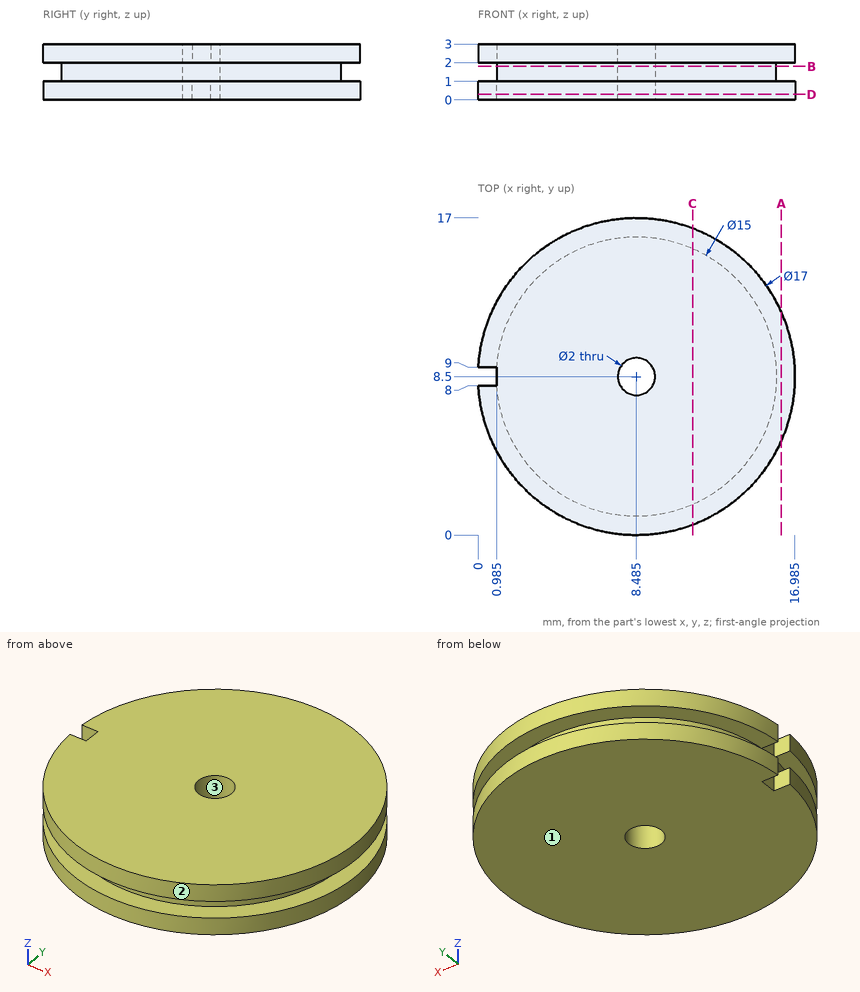
Geometry check sheet. Reference: drawing and pictorial views, mm from the part's lowest x, y, z. Round coordinates to 2 decimals unless told otherwise and drop trailing zeros. Order: outer loops, then holes, each group sorted by start corner. A loop starts at its lowest first (then second) coordinate and runs counter-clockwise, first axis right, second up. Notation, with made-up numbers: (-0.75, 54) - (56.25, 54) arc R29 ccw to (56.25, 86) - close; hole circle Ø3 at (15, 84). An arc over 180 degrees is marked (long way). Use a Markdown table: item, result. Add a question column.
1) Gauge pin test, flat ends, axial feed: P1, Ø1, axis at x = 6.5, z = 1, coming from the +Y side; P2, Ø1.1, axis at x = 0.5, z = 2.5, coming from the -Y side; P3, Ø0.8, axis at x = 0.5, z = 0.5, coming from the +Y side (1 decimal). Record the tip position at first contact, or that the pin passes through.
2) Section check C-C (x = 11.5). Record the cut outline in (y, z), then the cut area to 3 significant figures.
3) Section check B-B (z = 1.8). Record the cut outline in (x, y) (1 decimal), then the cut area to 3 significant figures.
4) Section check A-A (x = 16.25). Record the cut outline in (y, z).
5) Section check D-D (z = 0.3). Record the cut outline in (x, y) (1 decimal).
6) Mould release check, pull along Y, two halves, no side actions. Record for the marked faces 1, 2 and 3: released by +Y, released by -Y, zero draft, split by the parting line, or undercut.
7) Thickness scan on line 1 along Y through (x, z) = (8.5, 2.7); line 2 along Y through (x, z) = (14.25, 2.15) (1 decimal); line 3 along X through (y, z) = (14.75, 1.6). Record the ranges inside material, lowest first.
Established:
| question | item | result |
|---|---|---|
| 1 | P1 | y = 16.87 |
| 1 | P2 | y = 4.38 |
| 1 | P3 | y = 12.3 |
| 2 | outline | (0.55, 0) - (16.45, 0) - (16.45, 1) - (15.37, 1) - (15.37, 2) - (16.45, 2) - (16.45, 3) - (0.55, 3) - (0.55, 2) - (1.63, 2) - (1.63, 1) - (0.55, 1) - close |
| 2 | area | 45.5 mm2 |
| 3 | outline | circle Ø15 at (8.5, 8.5); hole circle Ø2 at (8.5, 8.5) |
| 3 | area | 174 mm2 |
| 4 | outline | (5.04, 0) - (11.96, 0) - (11.96, 1) - (5.04, 1) - close; (5.04, 2) - (11.96, 2) - (11.96, 3) - (5.04, 3) - close |
| 5 | outline | (0, 8) arc R8.5 ccw (long way) to (0, 9) - (1, 9) - (1, 8) - close; hole circle Ø2 at (8.5, 8.5) |
| 6 | face 1 | zero draft |
| 6 | face 2 | split by the parting line |
| 6 | face 3 | undercut |
| 7 | line 1 | 0 to 7.5, 9.5 to 17 |
| 7 | line 2 | 2.3 to 14.7 |
| 7 | line 3 | 4.34 to 12.63 |
